Model file for the job. Use its own axes, mm. A direction names the side the tool comes from. Give positions to 0.01 mm unless a question says otherwise; leave off trailing zeros. Order: outer loops, then holes, each group sorted by start corner. A loop starts at its lowest first (then second) coordinate and runs counter-clockwise, first axis right, second up. Notation, with made-up numbers: (88, 36.25) -> (111, 36.25) arc R27 ccw to (111, 62.25) -> close; hole circle Ø9 at (36.25, -12). An arc over 180 degrees is marked (long way). Use CSV: the item, a comma, the result in double quotes. Start each with the question number.
1. Drop flat-ended pins along their axis: pin 1 (1 mm diameter, centred on y = 27.5, z = 33.5, fed in from +X); pin 2 (16 mm diameter, centred on x = 67, z = -15.5, fed in from +Y); pin 3 (2 mm diameter, centred on x = 115.91, z = -5.23, fed in from -Y); pin 4 (2 mm diameter, centred on x = 68, y = 57, fed in from +Z). Give the stop position or say it passes through.
2. Cut at C-C on z = 10.5. List the corners of the cut face in (x, y).
3. Wall check: line 1 (Z direction, x = 83, y = 8); line 2 (X direction, y = 9, z = 106); line 3 (X direction, y = 19.5, z = -6). Give the ranges that are in metal, low to high. Write a range as from..to.
4. Pull direction X, two halves, no side cores. Call faces 5 (the flat face through (-46.593, 8, 115)), 6 (the flat face through (130.907, 9, -20)), 7 (the cylindrical face through (-56.628, 98.142, 86.274)): released by +X, released by -X, zero draft, split by the parting line, or undercut.
5. Cut at A-A on x = 61. List the corners of the cut face in (y, z).
6. Cut at B-B on y = 23. List the corners of the cut face in (x, z).
7. 3-axis set-ups, long thin cutter, end or side, ignore diameter. For faces 1 (the flat face through (40.907, 8, -5)), 2 (the flat face through (-34, 18, -5.23)), 3 (the flat face through (-46.593, 18, -15)), 4 (the flat face through (7.3, 70, -25.5)): which of +Z, -Z, +X, -X, +Y, -Y reach the whole face in a straight line?
8. Cut at D-D on y = 79. List the corners of the cut face in (x, z), then the cut area to 3 significant figures.
```python
from build123d import *

# Parameters (mm, degrees)
BOSS_EXTRUDE1_DEPTH = 10
SKETCH2_W           = 90
SKETCH2_H           = 25
SKETCH2_W_2         = 25
SKETCH2_H_2         = 90
CUT_EXTRUDE1_DEPTH  = 5
SKETCH3_R           = 1.65
CUT_EXTRUDE2_DEPTH  = 6
SKETCH4_W           = 25
SKETCH4_H           = 25
BOSS_EXTRUDE2_DEPTH = 22
SKETCH5_R           = 4
CUT_EXTRUDE3_DEPTH  = 191
FILLET1_R           = 5
SKETCH6_W           = 190
SKETCH6_H           = 90
BOSS_EXTRUDE3_DEPTH = 5
SKETCH7_R           = 4
SKETCH7_R_2         = 12.5
SKETCH7_R_3         = 1.65
CUT_EXTRUDE4_DEPTH  = 6
SKETCH8_W           = 185
SKETCH8_H           = 5
BOSS_EXTRUDE4_DEPTH = 60
SKETCH9_R           = 4
CUT_EXTRUDE5_DEPTH  = 191
CUT_EXTRUDE6_DEPTH  = 6
FILLET2_R           = 10
SKETCH11_W          = 50
SKETCH11_H          = 25
CUT_EXTRUDE7_DEPTH  = 1
SKETCH12_R          = 1.65
CUT_EXTRUDE8_DEPTH  = 5
SKETCH13_W          = 50
SKETCH13_H          = 25
CUT_EXTRUDE9_DEPTH  = 1
SKETCH14_R          = 1.65
CUT_EXTRUDE10_DEPTH = 5


with BuildPart() as part:
    # Sketch1 → Boss-Extrude1 (new body)
    with BuildSketch(Plane(origin=(0, 0, 0), x_dir=(1, 0, 0), z_dir=(0, 1, 0))):
        with BuildLine():
            Line((-59.092867484, 30.230027325), (130.907132516, 30.230027325))
            Line((130.907132516, 30.230027325), (130.907132516, -19.769972675))
            Line((130.907132516, -19.769972675), (0.907132516, -19.769972675))
            ThreePointArc((0.907132516, -19.769972675), (-6.163935296, -22.698904864), (-9.092867484, -29.769972675))
            Line((-9.092867484, -29.769972675), (-9.092867484, -159.769972675))
            Line((-9.092867484, -159.769972675), (-59.092867484, -159.769972675))
            Line((-59.092867484, -159.769972675), (-59.092867484, 30.230027325))
        make_face()
    extrude(amount=BOSS_EXTRUDE1_DEPTH)

    # Sketch2 → Cut-Extrude1 (cut)
    with BuildSketch(Plane(origin=(0, 10, 0), x_dir=(1, 0, 0), z_dir=(0, 1, 0))):
        with Locations((85.907132516, 5.230027325)):
            Rectangle(SKETCH2_W, SKETCH2_H)
        with Locations((-34.092867484, -114.769972675)):
            Rectangle(SKETCH2_W_2, SKETCH2_H_2)
    extrude(amount=-CUT_EXTRUDE1_DEPTH, mode=Mode.SUBTRACT)

    # Sketch3 → Cut-Extrude2 (cut, through all)
    with BuildSketch(Plane(origin=(0, 5, 0), x_dir=(1, 0, 0), z_dir=(0, 1, 0))):
        with Locations((55.907132516, 5.230027325)):
            Circle(SKETCH3_R)
        with Locations((115.907132516, 5.230027325)):
            Circle(SKETCH3_R)
        with Locations((-34.092867483, -84.769972675)):
            Circle(SKETCH3_R)
        with Locations((-34.092867483, -144.769972675)):
            Circle(SKETCH3_R)
    extrude(amount=-CUT_EXTRUDE2_DEPTH, mode=Mode.SUBTRACT)

    # Sketch4 → Boss-Extrude2 (add)
    with BuildSketch(Plane(origin=(0, 10, 0), x_dir=(1, 0, 0), z_dir=(0, 1, 0))):
        with Locations((-34.092867484, 17.730027325)):
            Rectangle(SKETCH4_W, SKETCH4_H)
    extrude(amount=BOSS_EXTRUDE2_DEPTH)

    # Sketch5 → Cut-Extrude3 (cut, through all)
    with BuildSketch(Plane(origin=(0, 0, -30.230027325), x_dir=(-1, 0, 0), z_dir=(0, 0, -1))):
        with Locations((34.092867484, 23)):
            Circle(SKETCH5_R)
    extrude(amount=-CUT_EXTRUDE3_DEPTH, mode=Mode.SUBTRACT)

    # Fillet1
    fillet1_edges = [part.edges().sort_by_distance(p)[0] for p in [
        (-46.592867484, 32, -17.730027325),
        (-21.592867484, 32, -17.730027325),
    ]]
    fillet(fillet1_edges, radius=FILLET1_R)

    # Sketch6 → Boss-Extrude3 (add)
    with BuildSketch(Plane.ZY.offset(59.092867484)):
        with Locations((64.769972675, 55)):
            Rectangle(SKETCH6_W, SKETCH6_H)
    extrude(amount=-BOSS_EXTRUDE3_DEPTH)

    # Sketch7 → Cut-Extrude4 (cut, through all)
    with BuildSketch(Plane(origin=(-54.092867484, 0, 0), x_dir=(0, 0, -1), z_dir=(1, 0, 0))):
        with Locations((10.230027325, 62)):
            Circle(SKETCH7_R)
        with Locations((-63.970957781, 79)):
            Circle(SKETCH7_R_2)
        with Locations((-79.470957781, 94.5)):
            Circle(SKETCH7_R_3)
        with Locations((-48.470957781, 94.5)):
            Circle(SKETCH7_R_3)
        with Locations((-48.470957781, 63.5)):
            Circle(SKETCH7_R_3)
        with Locations((-79.470957781, 63.5)):
            Circle(SKETCH7_R_3)
    extrude(amount=-CUT_EXTRUDE4_DEPTH, mode=Mode.SUBTRACT)

    # Sketch8 → Boss-Extrude4 (add)
    with BuildSketch(Plane(origin=(0, 10, 0), x_dir=(1, 0, 0), z_dir=(0, 1, 0))):
        with Locations((38.407132516, 27.730027325)):
            Rectangle(SKETCH8_W, SKETCH8_H)
    extrude(amount=BOSS_EXTRUDE4_DEPTH)

    # Sketch9 → Cut-Extrude5 (cut, through all)
    with BuildSketch(Plane(origin=(0, 0, -30.230027325), x_dir=(-1, 0, 0), z_dir=(0, 0, -1))):
        with Locations((34.092867484, 23)):
            Circle(SKETCH9_R)
    extrude(amount=-CUT_EXTRUDE5_DEPTH, mode=Mode.SUBTRACT)

    # Sketch10 → Cut-Extrude6 (cut, through all)
    with BuildSketch(Plane(origin=(-54.092867484, 0, 0), x_dir=(0, 0, -1), z_dir=(1, 0, 0))):
        Polygon((-159.769972675, 70), (-98.390064809, 70), (-87.470957781, 100), (-159.769972675, 100), align=None)
        Polygon((-40.470957781, 100), (-29.551850753, 70), (25.230027325, 70), (30.230027325, 70), (30.230027325, 100), align=None)
    extrude(amount=-CUT_EXTRUDE6_DEPTH, mode=Mode.SUBTRACT)

    # Fillet2
    fillet2_edges = [part.edges().sort_by_distance(p)[0] for p in [
        (-56.592867484, 100, 87.470957781),
        (-56.592867484, 70, 98.390064809),
        (-56.592867484, 100, 40.470957781),
        (-56.592867484, 70, 29.551850753),
    ]]
    fillet(fillet2_edges, radius=FILLET2_R)

    # Sketch11 → Cut-Extrude7 (cut)
    with BuildSketch(Plane.XY.offset(-25.230027325)):
        with Locations((105.907132516, 57.5)):
            Rectangle(SKETCH11_W, SKETCH11_H)
    extrude(amount=-CUT_EXTRUDE7_DEPTH, mode=Mode.SUBTRACT)

    # Sketch12 → Cut-Extrude8 (cut, through all)
    with BuildSketch(Plane.XY.offset(-26.230027325)):
        with Locations((90.907132516, 57.5)):
            Circle(SKETCH12_R)
        with Locations((120.907132516, 57.5)):
            Circle(SKETCH12_R)
    extrude(amount=-CUT_EXTRUDE8_DEPTH, mode=Mode.SUBTRACT)

    # Sketch13 → Cut-Extrude9 (cut)
    with BuildSketch(Plane(origin=(-54.092867484, 0, 0), x_dir=(0, 0, -1), z_dir=(1, 0, 0))):
        with Locations((-134.769972675, 57.5)):
            Rectangle(SKETCH13_W, SKETCH13_H)
    extrude(amount=-CUT_EXTRUDE9_DEPTH, mode=Mode.SUBTRACT)

    # Sketch14 → Cut-Extrude10 (cut, through all)
    with BuildSketch(Plane(origin=(-55.092867484, 0, 0), x_dir=(0, 0, -1), z_dir=(1, 0, 0))):
        with Locations((-149.769972675, 57.5)):
            Circle(SKETCH14_R)
        with Locations((-119.769972675, 57.5)):
            Circle(SKETCH14_R)
    extrude(amount=-CUT_EXTRUDE10_DEPTH, mode=Mode.SUBTRACT)


solid = part.part
```
Verdict:
1,pin 1,"x = -54.09"
1,pin 2,"y = 10"
1,pin 3,"through"
1,pin 4,"z = -25.23"
2,outline,"(-59.09, 0) -> (130.91, 0) -> (130.91, 10) -> (-54.09, 10) -> (-54.09, 70) -> (-59.09, 70) -> close"
3,line 1,"-30.23..-17.73, 7.27..19.77"
3,line 2,"-59.09..-46.59, -21.59..-9.09"
3,line 3,"-59.09..-54.09, -46.59..-36.03, -32.16..-21.59"
4,face 5,"undercut"
4,face 6,"released by +X"
4,face 7,"zero draft"
5,outline,"(0, -30.23) -> (70, -30.23) -> (70, -25.23) -> (10, -25.23) -> (10, -17.73) -> (5, -17.73) -> (5, 7.27) -> (10, 7.27) -> (10, 19.77) -> (0, 19.77) -> close"
6,outline,"(-59.09, -30.23) -> (-38.09, -30.23) -> (-38.09, -5.23) -> (-46.59, -5.23) -> (-46.59, -25.23) -> (-54.09, -25.23) -> (-54.09, 159.77) -> (-59.09, 159.77) -> close; (-30.09, -30.23) -> (130.91, -30.23) -> (130.91, -25.23) -> (-21.59, -25.23) -> (-21.59, -5.23) -> (-30.09, -5.23) -> close"
7,face 1,"+X, +Y"
7,face 2,"+Z, +X, +Y"
7,face 3,"+Z, +Y"
7,face 4,"-Z, +X, -X, +Y"
8,outline,"(-59.09, 32.83) -> (-54.09, 32.83) -> (-54.09, 51.47) -> (-59.09, 51.47) -> close; (-59.09, 76.47) -> (-54.09, 76.47) -> (-54.09, 95.11) -> (-59.09, 95.11) -> close"
8,area,"186 mm^2"
